Geometry check sheet. Reference: the model listing, model coordinates, mm. A direction names the side the tool comes from. Coordinates: 2 decimals unless noted, no trailing zeros. Loops run counter-clockwise (first coordinate to the right, second up) from the corner with the lowest first, then second, coordinate; pieces in that order, holes last.
from build123d import *

# Parameters (mm, degrees)
BOSS_EXTRUDE1_DEPTH     = 12.7
BOSS_EXTRUDE2_DEPTH     = 38.1
FILLET1_R               = 25.4
FILLET2_R               = 20.32
FILLET3_R               = 6.35
FILLET4_R               = 1.2699999999999994
CUT_EXTRUDE5_REACH      = 82.133
CUT_EXTRUDE5_END_RADIUS = 25.400000000000002
SKETCH6_R               = 3.4289999999999985
CUT_EXTRUDE6_REACH      = 77.736
CUT_EXTRUDE6_END_RADIUS = 25.400000000000002
SKETCH7_R               = 5.55625
SKETCH7_R_2             = 5.556250000000004


with BuildPart() as part:
    # Sketch1 → Boss-Extrude1 (new body)
    with BuildSketch(Plane(origin=(0, 0, 0), x_dir=(1, 0, 0), z_dir=(0, 1, 0))):
        Polygon((39.86388888888888, 22.225000000000012), (-39.86388888888888, 22.225), (-28.574999999999996, -28.57499999999998), (28.575000000000006, -28.574999999999978), align=None)
        Polygon((41.27499999999999, 28.575000000000014), (-41.275000000000006, 28.575000000000003), (-39.863888888888894, 22.225), (39.86388888888888, 22.225000000000012), align=None)
    extrude(amount=BOSS_EXTRUDE1_DEPTH)

    # Sketch1<5> → Boss-Extrude2 (add)
    with BuildSketch(Plane(origin=(0, 0, 0), x_dir=(1, 0, 0), z_dir=(0, 1, 0))):
        Polygon((41.27499999999999, 28.575000000000014), (-41.275000000000006, 28.575000000000003), (-39.863888888888894, 22.225), (39.86388888888888, 22.225000000000012), align=None)
    extrude(amount=BOSS_EXTRUDE2_DEPTH)

    # Fillet1
    fillet1_edges = [part.edges().sort_by_distance(p)[0] for p in [
        (0, 12.7, -22.22500000000001),
    ]]
    fillet(fillet1_edges, radius=FILLET1_R - 0.0001)  # a hair under: the kernel refuses the full size

    # Fillet2
    fillet2_edges = [part.edges().sort_by_distance(p)[0] for p in [
        (28.575000000000006, 6.35, 28.574999999999978),
        (-28.574999999999996, 6.35, 28.57499999999998),
    ]]
    fillet(fillet2_edges, radius=FILLET2_R)

    # Fillet3
    fillet3_edges = [part.edges().sort_by_distance(p)[0] for p in [
        (-7.11e-15, 0, -28.57500000000001),
    ]]
    fillet(fillet3_edges, radius=FILLET3_R)

    # Fillet4
    fillet4_edges = [part.edges().sort_by_distance(p)[0] for p in [
        (0, 38.1, -22.22500000000001),
        (-7.11e-15, 38.1, -28.57500000000001),
    ]]
    fillet(fillet4_edges, radius=FILLET4_R)

    # Cut-Extrude5: up to this cylinder (the profile starts outside it)
    cut_extrude5_end = Plane(origin=(3.97e-15, 38.1, 3.1749999999999905), z_dir=(-1, 0, 1.3e-16)) * Cylinder(CUT_EXTRUDE5_END_RADIUS, 254.166, mode=Mode.PRIVATE)
    # Sketch6 → Cut-Extrude5 (cut, up to the surface)
    with BuildSketch(Plane(origin=(-3.6e-15, 0, -28.57500000000001), x_dir=(-1, 0, 1.3e-16), z_dir=(-1.3e-16, 0, -1)), mode=Mode.PRIVATE) as cut_extrude5_sk1:
        with Locations((-19.05, 28.701999999999998)):
            Circle(SKETCH6_R)
    cut_extrude5_tool1 = extrude(cut_extrude5_sk1.sketch, amount=-CUT_EXTRUDE5_REACH, mode=Mode.PRIVATE) - cut_extrude5_end
    add(cut_extrude5_tool1.solids().sort_by_distance((19.05, 28.702, -28.575))[0], mode=Mode.SUBTRACT)
    # Sketch6 → Cut-Extrude5 (cut, up to the surface)
    with BuildSketch(Plane(origin=(-3.6e-15, 0, -28.57500000000001), x_dir=(-1, 0, 1.3e-16), z_dir=(-1.3e-16, 0, -1)), mode=Mode.PRIVATE) as cut_extrude5_sk2:
        with Locations((19.05, 28.701999999999998)):
            Circle(SKETCH6_R)
    cut_extrude5_tool2 = extrude(cut_extrude5_sk2.sketch, amount=-CUT_EXTRUDE5_REACH, mode=Mode.PRIVATE) - cut_extrude5_end
    add(cut_extrude5_tool2.solids().sort_by_distance((-19.05, 28.702, -28.575))[0], mode=Mode.SUBTRACT)

    # Cut-Extrude6: up to this cylinder (the profile starts outside it)
    cut_extrude6_end = Plane(origin=(3.97e-15, 38.1, 3.1749999999999905), z_dir=(-1, 0, 1.3e-16)) * Cylinder(CUT_EXTRUDE6_END_RADIUS, 245.372, mode=Mode.PRIVATE)
    # Sketch7 → Cut-Extrude6 (cut, up to the surface)
    with BuildSketch(Plane(origin=(-2.8e-15, 0, -22.22500000000001), x_dir=(-1, 0, 1.3e-16), z_dir=(-1.3e-16, 0, -1)), mode=Mode.PRIVATE) as cut_extrude6_sk1:
        with Locations((-19.05, 28.701999999999998)):
            Circle(SKETCH7_R)
    cut_extrude6_tool1 = extrude(cut_extrude6_sk1.sketch, amount=-CUT_EXTRUDE6_REACH, mode=Mode.PRIVATE) - cut_extrude6_end
    add(cut_extrude6_tool1.solids().sort_by_distance((19.05, 28.702, -22.225))[0], mode=Mode.SUBTRACT)
    # Sketch7 → Cut-Extrude6 (cut, up to the surface)
    with BuildSketch(Plane(origin=(-2.8e-15, 0, -22.22500000000001), x_dir=(-1, 0, 1.3e-16), z_dir=(-1.3e-16, 0, -1)), mode=Mode.PRIVATE) as cut_extrude6_sk2:
        with Locations((19.05, 28.701999999999998)):
            Circle(SKETCH7_R_2)
    cut_extrude6_tool2 = extrude(cut_extrude6_sk2.sketch, amount=-CUT_EXTRUDE6_REACH, mode=Mode.PRIVATE) - cut_extrude6_end
    add(cut_extrude6_tool2.solids().sort_by_distance((-19.05, 28.702, -22.225))[0], mode=Mode.SUBTRACT)


solid = part.part
(1) Gauge pin test, flat ends, axial feed: pin 1 Ø5.5 at (x, y) = (-17.5, 29) entering from +Z (3 decimals); pin 2 Ø3 at (x, z) = (2, 15.5) entering from +Y; pin 3 Ø1 at (y, z) = (10.5, 0.5) entering from -X (3 decimals); pin 4 Ø9 at (x, y) = (19.05, 28.702) entering from -Z (3 decimals). Record the tip position at first contact, or that the pin passes through.
Findings:
pin 1: stops at z = -22.225
pin 2: stops at y = 12.7
pin 3: stops at x = -34.925
pin 4: stops at z = -28.575
(2) Sectioned sample at A-A on y = 15. Record the cut outline in (x, z) (3 decimals), and give its area (3 significant figures).
Findings:
outline: (-41.275, -28.575) - (41.275, -28.575) - (36.567, -7.387) - (-36.567, -7.387) - close
area: 1,650 mm2
(3) Draft check along X on faces 4 (the cylindrical face through (24.839, 6.439, 24.225)), 5 (the flat face through (-37.775, 10.317, -12.827)), 6 (the flat face through (22, 26, -22.225)), 7 (the flat face through (-1, 38.1, -25)). Enter one of: +X half, -X half, draft (parallel to the pull), parting line (faces both ways), or undercut.
Findings:
face 4: +X half
face 5: -X half
face 6: undercut
face 7: draft
(4) Sectioned sample at B-B on z = 0.5. Record the cut outline in (x, y), and give its area (3 significant figures).
Findings:
outline: (-34.81, 0) - (34.81, 0) - (34.81, 12.84) - (-34.81, 12.84) - close
area: 894 mm2
(5) Scan lines: L1, parallel to Y at x = -32.5, z = 5; L2, parallel to Y at x = 19.05, z = -26.5; L3, parallel to Y at x = -19.05, z = -25.5. Record each from-to range of solid material in increasing order.
Findings:
L1: y = 0 to 12.7
L2: y = 1.65 to 25.27, 32.13 to 38.1
L3: y = 0.91 to 25.27, 32.13 to 38.1
(6) Access from +Z, -Z, +X, -X, +Y, -Y to the whole of each face (thin tool, end or side, straight path). Record for faces 1 (the cylindrical face through (-22.32, 29.73, -25.44)), 2 (the flat face through (0, 12.7, 16)), 3 (the cylindrical face through (-17.846, 23.278, -20.357)).
Findings:
face 1: +Z, -Z
face 2: +Z, +X, -X, +Y
face 3: +Z
